```python
from build123d import *

# Parameters (mm, degrees)
SKETCH1_R           = 3
SKETCH1_W           = 33
SKETCH1_H           = 80
BOSS_EXTRUDE1_DEPTH = 4
SKETCH4_R           = 2
CUT_EXTRUDE2_DEPTH  = 10
SKETCH5_R           = 2
CUT_EXTRUDE3_DEPTH  = 10


with BuildPart() as part:
    # Sketch1 → Boss-Extrude1 (new body)
    with BuildSketch(Plane.XY):
        Polygon((-145, -20.635083269), (-145, -55), (145, -55), (145, -20.635083269), (145, 40), (145, 55), (-145, 55), (-145, 40), align=None)
        with Locations((-108, -45)):
            Circle(SKETCH1_R, mode=Mode.SUBTRACT)
        with Locations((-125, 47)):
            Circle(SKETCH1_R, mode=Mode.SUBTRACT)
        with Locations(Location((125, 47, 0), (0, 0, 180))):
            Circle(SKETCH1_R, mode=Mode.SUBTRACT)
        with Locations(Location((108, -45, 0), (0, 0, 180))):
            Circle(SKETCH1_R, mode=Mode.SUBTRACT)
        with Locations((-120.5, 0)):
            Rectangle(SKETCH1_W, SKETCH1_H, mode=Mode.SUBTRACT)
        Polygon((-68, -30), (-38, -30), (-38, -20), (-4.5, -20), (-4.5, 20), (-38, 20), (-38, 30), (-68, 30), align=None, mode=Mode.SUBTRACT)
        Polygon((38, 20), (38, 30), (68, 30), (68, -30), (38, -30), (38, -20), (4.5, -20), (4.5, 20), align=None, mode=Mode.SUBTRACT)
        with Locations((120.5, 0)):
            Rectangle(SKETCH1_W, SKETCH1_H, mode=Mode.SUBTRACT)
    extrude(amount=BOSS_EXTRUDE1_DEPTH)

    # Sketch4 → Cut-Extrude2 (cut)
    with BuildSketch(Plane(origin=(0, 0, 0), x_dir=(-1, 0, 0), z_dir=(0, 0, -1))):
        with Locations((-141.5, 0)):
            Circle(SKETCH4_R)
    cut_extrude2 = extrude(amount=-CUT_EXTRUDE2_DEPTH, mode=Mode.SUBTRACT)

    # Sketch5 → Cut-Extrude3 (cut)
    with BuildSketch(Plane(origin=(0, 0, 0), x_dir=(-1, 0, 0), z_dir=(0, 0, -1))):
        with Locations((-78.5, 0)):
            Circle(SKETCH5_R)
    cut_extrude3 = extrude(amount=-CUT_EXTRUDE3_DEPTH, mode=Mode.SUBTRACT)

    # Mirror1: Cut-Extrude2, Cut-Extrude3 across plane
    add(cut_extrude2.mirror(Plane.ZY), mode=Mode.SUBTRACT)
    add(cut_extrude3.mirror(Plane.ZY), mode=Mode.SUBTRACT)


solid = part.part
```
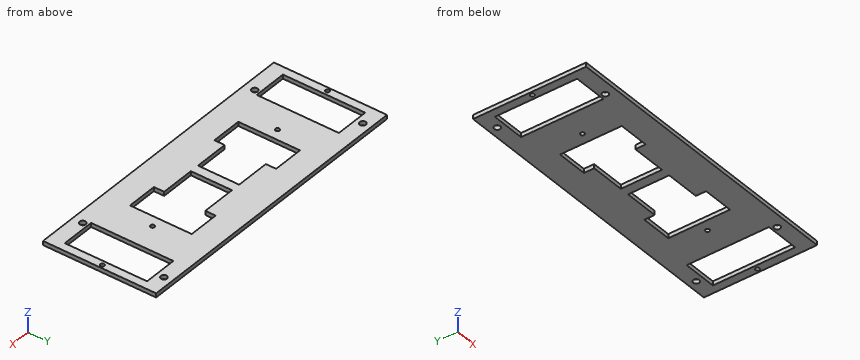
Work out the finished part from the listing and answer in its coordinate system (mm). Coordinates: 2 decimals unless noted, no trailing zeros. Loops run counter-clockwise (first coordinate to the right, second up) from the corner with the lowest first, then second, coordinate; pieces in that order, holes last. Notation, with made-up numbers: (-18, -15.75) - (18, -15.75) arc R20 ccw to (18, -4.75) - close; hole circle Ø4 at (13.25, -39). An arc over 180 degrees is marked (long way). Use a Markdown table: item, result.
Item 1: Find section D-D, the plane y = 7.5. Determine the outline of the cut face in (x, z).
Evaluation:
| item | result |
|---|---|
| outline | (-145, 0) - (-137, 0) - (-137, 4) - (-145, 4) - close; (-104, 0) - (-68, 0) - (-68, 4) - (-104, 4) - close; (-4.5, 0) - (4.5, 0) - (4.5, 4) - (-4.5, 4) - close; (68, 0) - (104, 0) - (104, 4) - (68, 4) - close; (137, 0) - (145, 0) - (145, 4) - (137, 4) - close |
Item 2: Find section B-B, the plane x = -125. Determine the outline of the cut face in (y, z), and give its area (3 significant figures).
Evaluation:
| item | result |
|---|---|
| outline | (-55, 0) - (-40, 0) - (-40, 4) - (-55, 4) - close; (40, 0) - (44, 0) - (44, 4) - (40, 4) - close; (50, 0) - (55, 0) - (55, 4) - (50, 4) - close |
| area | 96.0 mm2 |
Item 3: Given pin 1 Ø12 at (x, y) = (-9, 4.5) entering from -Z; pin 2 Ø3 at (x, y) = (-141.5, 0) entering from -Z, each flat-ended and moving along its own axis, determine where each tip first touches the part or whether it passes through.
Evaluation:
| item | result |
|---|---|
| pin 1 | stops at z = 0 |
| pin 2 | passes through |
Item 4: Find section C-C, the plane x = -32.5. Determine the outline of the cut face in (y, z).
Evaluation:
| item | result |
|---|---|
| outline | (-55, 0) - (-20, 0) - (-20, 4) - (-55, 4) - close; (20, 0) - (55, 0) - (55, 4) - (20, 4) - close |
Item 5: Find section A-A, the plane y = 47. Determine the outline of the cut face in (x, z).
Evaluation:
| item | result |
|---|---|
| outline | (-145, 0) - (-128, 0) - (-128, 4) - (-145, 4) - close; (-122, 0) - (122, 0) - (122, 4) - (-122, 4) - close; (128, 0) - (145, 0) - (145, 4) - (128, 4) - close |
Item 6: Consider probe 1 along X at (y, z) = (-26, 3.1); probe 2 along X at (y, z) = (-15, 3.75); probe 3 along Y at (x, z) = (-108, 1.5). Determine where each line is inside the solid, lowest interval first. Write a range as from..to.
Evaluation:
| item | result |
|---|---|
| probe 1 | x = -145..-137, -104..-68, -38..38, 68..104, 137..145 |
| probe 2 | x = -145..-137, -104..-68, -4.5..4.5, 68..104, 137..145 |
| probe 3 | y = -55..-48, -42..-40, 40..55 |
